```python
from build123d import *

# Parameters (mm, degrees)
CROQUIS1_R              = 5
SALIENTE_EXTRUIR1_DEPTH = 5
CROQUIS2_R              = 1.7
CORTAR_EXTRUIR1_DEPTH   = 5
CROQUIS3_R              = 2.95
CORTAR_EXTRUIR2_DEPTH   = 3
SALIENTE_EXTRUIR2_DEPTH = 3.25
CROQUIS5_R              = 1.7
CORTAR_EXTRUIR3_DEPTH   = 10
CORTAR_EXTRUIR4_DEPTH   = 1.7
REDONDEO1_R             = 3
SALIENTE_EXTRUIR3_DEPTH = 2.5
SALIENTE_EXTRUIR4_DEPTH = 21.75


with BuildPart() as part:
    # Croquis1 → Saliente-Extruir1 (new body)
    with BuildSketch(Plane.XY):
        with BuildLine():
            Line((-7.200520814, 3.25), (-26, 3.25))
            Line((-26, 3.25), (-26, -3.25))
            Line((-26, -3.25), (-7.200520814, -3.25))
            ThreePointArc((-7.200520814, -3.25), (0, -7.9), (7.200520814, -3.25))
            Line((7.200520814, -3.25), (26, -3.25))
            Line((26, -3.25), (26, 3.25))
            Line((26, 3.25), (7.200520814, 3.25))
            ThreePointArc((7.200520814, 3.25), (0, 7.9), (-7.200520814, 3.25))
        make_face()
        Circle(CROQUIS1_R, mode=Mode.SUBTRACT)
    extrude(amount=SALIENTE_EXTRUIR1_DEPTH)

    # Croquis2 → Cortar-Extruir1 (cut)
    with BuildSketch(Plane.XY.offset(5)):
        with Locations((-11, 0)):
            Circle(CROQUIS2_R)
        with Locations((11, 0)):
            Circle(CROQUIS2_R)
    extrude(amount=-CORTAR_EXTRUIR1_DEPTH, mode=Mode.SUBTRACT)

    # Croquis3 → Cortar-Extruir2 (cut)
    with BuildSketch(Plane.XY.offset(5)):
        with Locations((-11, 0)):
            Circle(CROQUIS3_R)
        with Locations((11, 0)):
            Circle(CROQUIS3_R)
    extrude(amount=-CORTAR_EXTRUIR2_DEPTH, mode=Mode.SUBTRACT)

    # Croquis4 → Saliente-Extruir2 (add, symmetric)
    with BuildSketch(Plane(origin=(0, 0, 0), x_dir=(1, 0, 0), z_dir=(0, 1, 0))):
        with BuildLine():
            Line((-26, 0), (-20.6, 0))
            ThreePointArc((-20.6, 0), (-23.334154241, 1.186812342), (-26, 2.52))
            Line((-26, 2.52), (-26, 0))
        make_face()
    saliente_extruir2 = extrude(amount=SALIENTE_EXTRUIR2_DEPTH, both=True)

    # Croquis5 → Cortar-Extruir3 (cut)
    with BuildSketch(Plane.XY.offset(5)):
        with Locations((-16.2, 0)):
            Circle(CROQUIS5_R)
    cortar_extruir3 = extrude(amount=-CORTAR_EXTRUIR3_DEPTH, mode=Mode.SUBTRACT)

    # Croquis6 → Cortar-Extruir4 (cut)
    with BuildSketch(Plane(origin=(0, 0, 0), x_dir=(-1, 0, 0), z_dir=(0, 0, -1))):
        Polygon((19.55, 0), (17.875, 2.901185103), (14.525, 2.901185103), (12.85, 0), (14.525, -2.901185103), (17.875, -2.901185103), align=None)
    cortar_extruir4 = extrude(amount=-CORTAR_EXTRUIR4_DEPTH, mode=Mode.SUBTRACT)

    # Simetría2: Saliente-Extruir2, Cortar-Extruir3, Cortar-Extruir4 across plane
    add(saliente_extruir2.mirror(Plane(origin=(0, 0, 0), x_dir=(0, 0, 1), z_dir=(1, 0, 0))))
    add(cortar_extruir3.mirror(Plane(origin=(0, 0, 0), x_dir=(0, 0, 1), z_dir=(1, 0, 0))), mode=Mode.SUBTRACT)
    add(cortar_extruir4.mirror(Plane(origin=(0, 0, 0), x_dir=(0, 0, 1), z_dir=(1, 0, 0))), mode=Mode.SUBTRACT)

    # Redondeo1
    redondeo1_edges = [part.edges().sort_by_distance(p)[0] for p in [
        (-26, 3.25, 1.24),
        (26, 3.25, 1.24),
        (26, -3.25, 1.24),
        (-26, -3.25, 1.24),
    ]]
    fillet(redondeo1_edges, radius=REDONDEO1_R)

    # Croquis7 → Saliente-Extruir3 (add)
    with BuildSketch(Plane.XY.offset(5)):
        with BuildLine():
            Line((-15.100260407, -3.25), (-7.200520814, -3.25))
            ThreePointArc((-7.200520814, -3.25), (0, -7.9), (7.200520814, -3.25))
            Line((7.200520814, -3.25), (15.100260407, -3.25))
            Line((15.100260407, -3.25), (15.100260407, -25))
            Line((15.100260407, -25), (-15.100260407, -25))
            Line((-15.100260407, -25), (-15.100260407, -3.25))
        make_face()
    extrude(amount=-SALIENTE_EXTRUIR3_DEPTH)

    # Croquis8 → Saliente-Extruir4 (add)
    with BuildSketch(Plane.XZ.offset(25)):
        with BuildLine():
            Line((-15.100260407, 2.5), (-15.100260407, 2))
            ThreePointArc((-15.100260407, 2), (-13.952935396, 2.262304947), (-12.800260407, 2.5))
            Line((-12.800260407, 2.5), (-15.100260407, 2.5))
        make_face()
        with BuildLine():
            Line((15.100260407, 2.5), (12.800260407, 2.5))
            ThreePointArc((12.800260407, 2.5), (13.952935396, 2.262304947), (15.100260407, 2))
            Line((15.100260407, 2), (15.100260407, 2.5))
        make_face()
    extrude(amount=-SALIENTE_EXTRUIR4_DEPTH)


solid = part.part
```
Read the model definition and answer for the solid it produces. Units are mm, in the model's axes. A direction names the side the tool comes from. Give positions to 0.01 mm unless a question says otherwise; leave off trailing zeros. Order: outer loops, then holes, each group sorted by start corner. A loop starts at its lowest first (then second) coordinate and runs counter-clockwise, first axis right, second up. Notation, with made-up numbers: (31, 58.5) -> (75, 58.5) arc R33 ccw to (75, 93.5) -> close; hole circle Ø1 at (50, 26.5). An arc over 180 degrees is marked (long way). Write item = value, one per line.
1. Given pin 1 (1.5 mm diameter, centred on y = -12.5, z = 4, fed in from -X); pin 2 (6 mm diameter, centred on x = -1.5, y = 0, fed in from -Z); pin 3 (2 mm diameter, centred on x = 20, z = -0.5, fed in from -Y); pin 4 (5.5 mm diameter, centred on x = -11, y = 0, fed in from +Z), each flat-ended and moving along its own axis, determine where each tip first touches the part or whether it passes through.
Numbers:
pin_1 = -15.1
pin_2 = through
pin_3 = -3.25
pin_4 = 2
2. A cutting plane is placed at B-B, the plane z = -2. Write down the section's boundary in (x, y).
Numbers:
outline = (-26, -0.25) arc R3 ccw to (-25, -2.48) -> (-25, 2.48) arc R3 ccw to (-26, 0.25) -> close; (25, -2.48) arc R3 ccw to (26, -0.25) -> (26, 0.25) arc R3 ccw to (25, 2.48) -> close
3. For faces 4 (the face through (-5, 2, 0)), 5 (the face through (-13.947, 0.13, 3.521)), 6 (the face through (-1.08, -4.88, 2.46)), 7 (the face through (0, -14, 2.5)), 8 (the face through (18, 1, 1.7)), determine the directions among +Z, -Z, +X, -X, +Y, -Y from which every point of the face is accessible in a straight line to the end or side of a thin tool.
Numbers:
face_4 = -Z, +Y, -Y
face_5 = +Z
face_6 = +Z, -Z
face_7 = -Z, -Y
face_8 = -Z
4. A cutting plane is placed at A-A, the plane x = -16.2. Write down the section's boundary in (y, z), and give its area (3 significant figures).
Numbers:
outline = (-3.25, 0) -> (-2.9, 0) -> (-2.9, 1.7) -> (-1.7, 1.7) -> (-1.7, 5) -> (-3.25, 5) -> close; (1.7, 1.7) -> (2.9, 1.7) -> (2.9, 0) -> (3.25, 0) -> (3.25, 5) -> (1.7, 5) -> close
area = 11.4 mm²
5. Straight lines are drawn through the part: line 1 along Y through (x, z) = (-11, 3.2); line 2 along X through (y, z) = (-0.5, 3); line 3 along Y through (x, z) = (-11, 1.65). For each, find the intervals that lie inside material, in ascending order.
Numbers:
line_1 = -25 to -2.95, 2.95 to 3.25
line_2 = -25.99 to -17.82, -14.58 to -13.91, -8.09 to -4.97, 4.97 to 8.09, 13.91 to 14.58, 17.82 to 25.99
line_3 = -3.25 to -1.7, 1.7 to 3.25
6. A cutting plane is placed at C-C, the plane z = 4.5. Write down the section's boundary in (x, y).
Numbers:
outline = (-26, -0.25) arc R3 ccw to (-23, -3.25) -> (-15.1, -3.25) -> (-15.1, -25) -> (15.1, -25) -> (15.1, -3.25) -> (23, -3.25) arc R3 ccw to (26, -0.25) -> (26, 0.25) arc R3 ccw to (23, 3.25) -> (7.2, 3.25) arc R7.9 ccw to (-7.2, 3.25) -> (-23, 3.25) arc R3 ccw to (-26, 0.25) -> close; hole circle Ø3.4 at (-16.2, 0); hole circle Ø5.9 at (-11, 0); hole circle Ø10 at (0, 0); hole circle Ø5.9 at (11, 0); hole circle Ø3.4 at (16.2, 0)
7. A cutting plane is placed at D-D, the plane y = 4.5. Write down the section's boundary in (x, z), and give its area (3 significant figures).
Numbers:
outline = (-6.49, 0) -> (-2.18, 0) -> (-2.18, 5) -> (-6.49, 5) -> close; (2.18, 0) -> (6.49, 0) -> (6.49, 5) -> (2.18, 5) -> close
area = 43.1 mm²
8. The mould has two halves that part along X. Classify faces 1 (the face through (0, -25, 4)), 2 (the face through (25.14, 2.35, 1.29)), 3 (the face through (18.7, -1.47, 0.84)): +X half, -X half, draft (parallel to the pull), parting line (faces both ways), or undercut.
Numbers:
face_1 = draft
face_2 = +X half
face_3 = undercut
